Verification items for the finished model (mm, model axes). Give positions to 0.01 mm unless a question says otherwise; leave off trailing zeros. Order: outer loops, then holes, each group sorted by start corner. A loop starts at its lowest first (then second) coordinate and runs counter-clockwise, first axis right, second up. Notation, with made-up numbers: M -16,-6 L -9,-6 A7 ccw -9,7 Z; hole C 5,-21.5 d11. An arc over 180 degrees is marked long. Answer as a JSON object with one key per item and string values.
```python
from build123d import *

# Parameters (mm, degrees)
SKETCH1_W                   = 34.925
SKETCH1_H                   = 34.925
SKETCH1_R                   = 7.9502
CUBE_DEPTH                  = 34.925
SKETCH1_3_R                 = 7.9502
CUT_EXTRUDE1_DEPTH          = 61.491874454
CIRPATTERN2_COUNT           = 2
CIRPATTERN2_ANGLE           = 90
CIRPATTERN3_COPY_1_SKETCH_R = 7.9502
CIRPATTERN3_COPY_1_DEPTH    = 61.491874454
CIRPATTERN3_COPY_2_SKETCH_R = 7.9502
CIRPATTERN3_COPY_2_DEPTH    = 61.491874454


with BuildPart() as part:
    # Sketch1 → Cube (new body)
    # profile 1 of 2: a face of its own
    with BuildSketch(Plane(origin=(0, 0, 0), x_dir=(1, 0, 0), z_dir=(0, 1, 0))):
        with Locations((17.4625, 17.4625)):
            Rectangle(SKETCH1_W, SKETCH1_H)
        with Locations((17.4625, 17.4625)):
            Circle(SKETCH1_R, mode=Mode.SUBTRACT)
    # profile 2 of 2: a face of its own
    with BuildSketch(Plane(origin=(0, 0, 0), x_dir=(1, 0, 0), z_dir=(0, 1, 0))):
        with Locations((17.4625, 17.4625)):
            Circle(SKETCH1_R)
    extrude(amount=CUBE_DEPTH)

    # Sketch1_3 → Cut-Extrude1 (cut, through all)
    with BuildSketch(Plane(origin=(0, 0, 0), x_dir=(1, 0, 0), z_dir=(0, 1, 0))):
        with Locations(Location((17.4625, 17.4625, 0), (0, 0, 270))):
            Circle(SKETCH1_3_R)
    cut_extrude1 = extrude(amount=CUT_EXTRUDE1_DEPTH, mode=Mode.SUBTRACT)

    # CirPattern2: Cut-Extrude1 ×2 about axis
    cirpattern2_axis = Axis((-1.74625, 17.4625, -17.4625), (1, 0, 0))
    for i in range(1, CIRPATTERN2_COUNT):
        add(cut_extrude1.rotate(cirpattern2_axis, i * CIRPATTERN2_ANGLE / (CIRPATTERN2_COUNT - 1)), mode=Mode.SUBTRACT)

    # CirPattern3 copy 1 sketch → CirPattern3 copy 1 (cut, through all)
    with BuildSketch(Plane(origin=(0, 34.925, -34.925), x_dir=(0, -1, 0), z_dir=(0, 0, 1))):
        with Locations(Location((17.4625, 17.4625, 0), (0, 0, 270))):
            Circle(CIRPATTERN3_COPY_1_SKETCH_R)
    extrude(amount=CIRPATTERN3_COPY_1_DEPTH, mode=Mode.SUBTRACT)

    # CirPattern3 copy 2 sketch → CirPattern3 copy 2 (cut, through all)
    with BuildSketch(Plane(origin=(0, 34.925, 0), x_dir=(0, -1, 0), z_dir=(1, 0, 0))):
        with Locations(Location((17.4625, 17.4625, 0), (0, 0, 270))):
            Circle(CIRPATTERN3_COPY_2_SKETCH_R)
    extrude(amount=CIRPATTERN3_COPY_2_DEPTH, mode=Mode.SUBTRACT)


solid = part.part
```
Q1. Section check C-C on z = -32. Record the cut outline in (x, y) (1 decimal).
Resolved:
{"outline": "M 0,0 L 34.9,0 L 34.9,34.9 L 0,34.9 Z; hole C 17.5,17.5 d15.9"}
Q2. Section check A-A on y = 15.5. Record the cut outline in (x, z) (3 decimals).
Resolved:
{"outline": "M 0,-34.925 L 9.758,-34.925 L 9.758,-25.167 L 0,-25.167 Z; M 0,-9.758 L 9.758,-9.758 L 9.758,0 L 0,0 Z; M 25.167,-34.925 L 34.925,-34.925 L 34.925,-25.167 L 25.167,-25.167 Z; M 25.167,-9.758 L 34.925,-9.758 L 34.925,0 L 25.167,0 Z"}
Q3. Gauge pin test, flat end, axial feed: pin 1 Ø20.5 at (y, z) = (17.46, -17.46) entering from +X (3 decimals). Record the tip position at first contact, or that the pin passes through.
Resolved:
{"pin 1": "stops at x = 34.925"}
Q4. Material ranges on L1, parallel to X at y = 17.5, z = -4 (3 decimals); L2, parallel to Y at x = 15, z = -31.5 (3 decimals); L3, parallel to X at y = 3.5, z = -13.5 (3 decimals), recorded low to high.
Resolved:
{"L1": "x = 0 to 9.512, 25.413 to 34.925", "L2": "y = 0 to 9.903, 25.022 to 34.925", "L3": "x = 0 to 10.57, 24.355 to 34.925"}
Q5. Section check B-B on x = 19.5. Record the cut outline in (y, z) (3 decimals).
Resolved:
{"outline": "M 0,-34.925 L 9.778,-34.925 L 9.778,-25.147 L 0,-25.147 Z; M 0,-9.778 L 9.778,-9.778 L 9.778,0 L 0,0 Z; M 25.147,-34.925 L 34.925,-34.925 L 34.925,-25.147 L 25.147,-25.147 Z; M 25.147,-9.778 L 34.925,-9.778 L 34.925,0 L 25.147,0 Z"}
Q6. Release check for a two-part mould opening along Y. For faces 1 (the face through (17, 9, -34.925)), 2 (the face through (9, 0, -18)), 3 (the face through (30.24, 12.09, -23.32)), 4 (the face through (9, 34.925, -18)) record: +Y half, -Y half, draft (parallel to the pull), parting line (faces both ways), or undercut.
Resolved:
{"face 1": "draft", "face 2": "-Y half", "face 3": "undercut", "face 4": "+Y half"}
Q7. Section check D-D on x = 7. Record the cut outline in (y, z) (1 decimal).
Resolved:
{"outline": "M 0,-34.9 L 34.9,-34.9 L 34.9,0 L 0,0 Z; hole C 17.5,-17.5 d15.9"}
